For this review, take the finished solid that the model builds, in its own axes (mm). Face numbers are marked on the shaded views. Coordinates: 2 decimals unless noted, no trailing zeros. Loops run counter-clockwise (first coordinate to the right, second up) from the corner with the lowest first, then second, coordinate; pieces in that order, holes last. Notation, with made-up numbers: (-0.5, -0.75) - (37.5, -0.75) arc R29 cw to (37.5, 36.25) - close; hole circle Ø11 at (26.25, 40). An arc over 180 degrees is marked (long way). One line per item, written item: value. Start each with the question number.
1. Take a section at A-A, the plane y = -3.5. State the section outline as (x, z) points, and give its area (3 significant figures).
2. Take a section at B-B, the plane z = 21. State the section outline as (x, y) points.
3. To check wall thickness, follow line 1 (Z direction, x = 8, y = -41); line 2 (Z direction, x = 17, y = -25.5); line 3 (Z direction, x = 3.5, y = -18). State the ranges of each line that lie inside material, in increasing order. Write a range as from..to.
4. Take a section at D-D, the plane y = -44.5. Count the separate pieces of the cut face and the enclosed holes in it, and give its area (3 significant figures).
5. Insertion check: pin 1 (6 mm diameter, centred on x = -19.5, y = -13, fed in from -Z); pin 2 (5 mm diameter, centred on y = -34, z = 59.5, fed in from +X); pin 3 (0.5 mm diameter, centred on x = 29, z = 59, fed in from -Y); pin 4 (4 mm diameter, centred on y = -19, z = 52.5, fed in from +X). Each pin has a flat end and moves straight along its axis. Give the tip position at first contact, or say it passes through.
6. Take a section at C-C, the plane x = -21.5. State the section outline as (y, z) points, and give its area (3 significant figures).
7. The part is to be moulded in two halves that separate along Z. For the marked faces 1, 2 and 3, say which applies: released by +Z, released by -Z, zero draft, split by the parting line, or undercut.
```python
from build123d import *

# Parameters (mm, degrees)
F1_DEPTH = 53.12398
F2_W     = 23.9413073286
F2_H     = 22.4265204743
F3_ANGLE = 90
F4_R     = 2.54
F6_DEPTH = 53.1249801
F8_DEPTH = 25.71572


with BuildPart() as f1:
    # F0 (on Front) → F1 (new body)
    with BuildSketch(Plane.XZ):
        Polygon((29.051852704, 29.0388607975), (-29.5177362859, 29.53094244), (0, 0), align=None)
    extrude(amount=F1_DEPTH)

    # F2 (on face) → F3 (revolve)
    with BuildSketch(Plane(origin=(0.2460079132, 0, 29.2808776473), x_dir=(0.9999647079, 0, -0.0084013613), z_dir=(0.0084013613, 0, 0.9999647079))):
        with Locations((-0.2708197571, -25.872068014)):
            Rectangle(F2_W, F2_H)
    revolve(axis=Axis((-0.2329417909, -53.12398, 29.2849016188), (0.9999647079, 0, -0.0084013613)), revolution_arc=F3_ANGLE)

    # F4
    f4_edges = [f1.edges().sort_by_distance(p)[0] for p in [
        (12.040709, -41.782941, 40.523222),
        (12.173937, -25.924996, 56.380607),
        (11.945429, -25.872068, 29.182583),
        (12.174382, -53.12398, 56.433533),
        (0.298358, -53.12398, 67.746968),
        (-11.76608, -53.12398, 56.634673),
        (0.109944, -53.12398, 45.321239),
        (-11.766525, -25.924996, 56.581747),
        (-0.024802, -14.658808, 29.283153),
        (-11.899753, -41.782941, 40.724362),
        (-0.024802, -37.085328, 29.283153),
        (-11.995033, -25.872068, 29.383723),
    ]]
    fillet(f4_edges, radius=F4_R)

    # F5 (on face) → F6 (cut, through all)
    with BuildSketch(Plane.XZ.offset(53.12398)):
        Polygon((0.0008033687, 3.5921023586), (22.9688507095, 26.5498784535), (-23.3355659609, 26.9389123157), align=None)
    extrude(amount=-F6_DEPTH, mode=Mode.SUBTRACT)

    # F7 (on face) → F8 (join)
    with BuildSketch(Plane(origin=(11.699420996, 0, -0.0982945313), x_dir=(0, 1, 0), z_dir=(0.9999647079, 0, -0.0084013613))):
        with BuildLine():
            Line((-23.396522254, 31.8219110662), (-23.0236383706, 31.8219110662))
            ThreePointArc((-23.0236383706, 31.8219110662), (-31.7641793665, 50.6417116997), (-50.58398, 59.3822526955))
            Line((-50.58398, 59.3822526955), (-50.58398, 59.0093688122))
            Line((-50.58398, 59.0093688122), (-23.396522254, 31.8219110662))
        make_face()
    extrude(amount=F8_DEPTH)


solid = f1.part
```
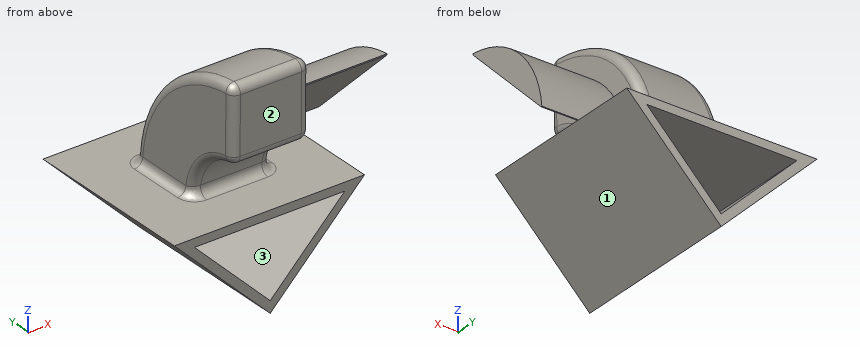
Solutions:
1. outline: (-29.52, 29.53) - (0, 0) - (29.05, 29.04) - close; hole (-23.34, 26.94) - (0, 3.59) - (22.97, 26.55) - close
1. area: 322 mm2
2. outline: (-20.99, -53.12) - (-17.4, -53.12) - (-17.4, 0) - (-20.99, 0) - close; (17.42, -53.12) - (21.01, -53.12) - (21.01, 0) - (17.42, 0) - close
3. line 1: 8..11.59, 26.68..29.22, 39.72..65.72
3. line 2: 16.99..20.58, 26.6..29.14, 33.78..41.36
3. line 3: 3.5..7.09, 26.71..44.93
4. separate pieces: 2
4. enclosed holes: 1
4. area: 1,030 mm2
5. pin 1: z = 16.51
5. pin 2: x = 12.21
5. pin 3: y = -50.58
5. pin 4: through
6. outline: (-53.12, 21.51) - (0, 21.51) - (0, 25.1) - (-53.12, 25.1) - close; (-53.12, 26.92) - (0, 26.92) - (0, 29.46) - (-53.12, 29.46) - close
6. area: 326 mm2
7. face 1: released by -Z
7. face 2: zero draft
7. face 3: undercut
